Could you check a few things on this model? Use its own coordinates, in mm. Give positions to 0.01 mm unless a question says otherwise; leave off trailing zeros. Loops run counter-clockwise (first coordinate to the right, second up) from the corner with the lowest first, then second, coordinate; pieces in that order, holes last. Notation, with made-up numbers: (2, 11.5) - (22, 11.5) arc R33 ccw to (22, 46.5) - close; hole circle Ø11 at (-10, 20.5). An arc over 180 degrees is marked (long way). Write each question's results on one line, items separated by ' | '. Start each with the question number.
1) If I drill on probe 1 along X at (y, z) = (1, -38.25); probe 2 along Z at (x, y) = (38.5, 3.45); probe 3 along X at (y, z) = (2.4, -18), over which ranges is the centre line in solid material (lowest first)? Write a range as [from, to].
2) I want a section at A-A, the plane z = 0. Write out the boundary of the cut face in (x, y).
3) I want a section at D-D, the plane y = 2.15. Count the separate pieces of the cut face and the enclosed holes in it, and give its area (3 significant figures).
4) I want a section at C-C, the plane x = 2. Write out the boundary of the cut face in (y, z).
5) I want a section at B-B, the plane z = -38.25. Write out the boundary of the cut face in (x, y), and give its area (3 significant figures).
6) If we mould it in two halves opening along X, with no side actions, what happens to faces 1 (the face through (-1, 5, -11)), 2 (the face through (15, 2, 0))? For each: +X half, -X half, draft (parallel to the pull), parting line (faces both ways), or undercut.
from build123d import *

# Parameters (mm, degrees)
SKETCH1_W               = 90
SKETCH1_H               = 90
SKETCH1_R               = 3.501345848
BOSS_EXTRUDE1_DEPTH     = 5
SKETCH2_R               = 1.75
SKETCH2_W               = 5
SKETCH2_H               = 10
CUT_EXTRUDE1_DEPTH      = 1
CUT_EXTRUDE1_DEPTH_BACK = 6
SKETCH3_R               = 4
CUT_EXTRUDE2_DEPTH      = 10


with BuildPart() as part:
    # Sketch1 → Boss-Extrude1 (new body)
    with BuildSketch(Plane(origin=(0, 0, 0), x_dir=(1, 0, 0), z_dir=(0, 1, 0))):
        Rectangle(SKETCH1_W, SKETCH1_H)
        Circle(SKETCH1_R, mode=Mode.SUBTRACT)
        with BuildLine():
            Line((-26.585786438, 19.514718626), (-14.489985056, 7.418917244))
            ThreePointArc((-14.489985056, 7.418917244), (-13.949056578, 6.425915745), (-14.033116428, 5.298267955))
            ThreePointArc((-14.033116428, 5.298267955), (-15, 0), (-14.033116428, -5.298267955))
            ThreePointArc((-14.033116428, -5.298267955), (-13.949056578, -6.425915745), (-14.489985056, -7.418917244))
            Line((-14.489985056, -7.418917244), (-26.585786438, -19.514718626))
            ThreePointArc((-26.585786438, -19.514718626), (-28.765366865, -19.948264128), (-30, -18.100505063))
            Line((-30, -18.100505063), (-30, 18.100505063))
            ThreePointArc((-30, 18.100505063), (-28.765366865, 19.948264128), (-26.585786438, 19.514718626))
        make_face(mode=Mode.SUBTRACT)
        with BuildLine():
            Line((-18.100505063, 30), (18.100505063, 30))
            ThreePointArc((18.100505063, 30), (19.948264128, 28.765366865), (19.514718626, 26.585786438))
            Line((19.514718626, 26.585786438), (7.418917244, 14.489985056))
            ThreePointArc((7.418917244, 14.489985056), (6.425915745, 13.949056578), (5.298267955, 14.033116428))
            ThreePointArc((5.298267955, 14.033116428), (0, 15), (-5.298267955, 14.033116428))
            ThreePointArc((-5.298267955, 14.033116428), (-6.425915745, 13.949056578), (-7.418917244, 14.489985056))
            Line((-7.418917244, 14.489985056), (-19.514718626, 26.585786438))
            ThreePointArc((-19.514718626, 26.585786438), (-19.948264128, 28.765366865), (-18.100505063, 30))
        make_face(mode=Mode.SUBTRACT)
        with BuildLine():
            Line((30, 18.100505063), (30, -18.100505063))
            ThreePointArc((30, -18.100505063), (28.765366865, -19.948264128), (26.585786438, -19.514718626))
            Line((26.585786438, -19.514718626), (14.489985056, -7.418917244))
            ThreePointArc((14.489985056, -7.418917244), (13.949056578, -6.425915745), (14.033116428, -5.298267955))
            ThreePointArc((14.033116428, -5.298267955), (15, 0), (14.033116428, 5.298267955))
            ThreePointArc((14.033116428, 5.298267955), (13.949056578, 6.425915745), (14.489985056, 7.418917244))
            Line((14.489985056, 7.418917244), (26.585786438, 19.514718626))
            ThreePointArc((26.585786438, 19.514718626), (28.765366865, 19.948264128), (30, 18.100505063))
        make_face(mode=Mode.SUBTRACT)
        with BuildLine():
            Line((19.514718626, -26.585786438), (7.418917244, -14.489985056))
            ThreePointArc((7.418917244, -14.489985056), (6.425915745, -13.949056578), (5.298267955, -14.033116428))
            ThreePointArc((5.298267955, -14.033116428), (0, -15), (-5.298267955, -14.033116428))
            ThreePointArc((-5.298267955, -14.033116428), (-6.425915745, -13.949056578), (-7.418917244, -14.489985056))
            Line((-7.418917244, -14.489985056), (-19.514718626, -26.585786438))
            ThreePointArc((-19.514718626, -26.585786438), (-19.948264128, -28.765366865), (-18.100505063, -30))
            Line((-18.100505063, -30), (18.100505063, -30))
            ThreePointArc((18.100505063, -30), (19.948264128, -28.765366865), (19.514718626, -26.585786438))
        make_face(mode=Mode.SUBTRACT)
    extrude(amount=BOSS_EXTRUDE1_DEPTH)

    # Sketch2 → Cut-Extrude1 (cut, two sides)
    with BuildSketch(Plane(origin=(0, 5, 0), x_dir=(1, 0, 0), z_dir=(0, 1, 0))) as cut_extrude1_sk:
        with Locations((-30, -38.25)):
            Circle(SKETCH2_R)
        with Locations((30, -38.25)):
            Circle(SKETCH2_R)
        with Locations((30, 38.25)):
            Circle(SKETCH2_R)
        with Locations((-30, 38.25)):
            Circle(SKETCH2_R)
        with Locations((37.5, 25)):
            Rectangle(SKETCH2_W, SKETCH2_H)
        with Locations((37.5, -25)):
            Rectangle(SKETCH2_W, SKETCH2_H)
        with Locations((-37.5, -25)):
            Rectangle(SKETCH2_W, SKETCH2_H)
        with Locations((-37.5, 25)):
            Rectangle(SKETCH2_W, SKETCH2_H)
    extrude(amount=CUT_EXTRUDE1_DEPTH, mode=Mode.SUBTRACT)
    extrude(cut_extrude1_sk.sketch, amount=-CUT_EXTRUDE1_DEPTH_BACK, mode=Mode.SUBTRACT)

    # Sketch3 → Cut-Extrude2 (cut)
    with BuildSketch(Plane(origin=(0, 5, 0), x_dir=(1, 0, 0), z_dir=(0, 1, 0))):
        Circle(SKETCH3_R)
    extrude(amount=-CUT_EXTRUDE2_DEPTH, mode=Mode.SUBTRACT)


solid = part.part
Answers:
1) probe 1: x = [-45, -31.75], [-28.25, 28.25], [31.75, 45] | probe 2: z = [-45, -30], [-20, 20], [30, 45] | probe 3: x = [-45, -30], [-25.07, -10.93], [10.93, 25.07], [30, 45]
2) outline: (-45, 0) - (-30, 0) - (-30, 5) - (-45, 5) - close; (-15, 0) - (-4, 0) - (-4, 5) - (-15, 5) - close; (4, 0) - (15, 0) - (15, 5) - (4, 5) - close; (30, 0) - (45, 0) - (45, 5) - (30, 5) - close
3) separate pieces: 1 | enclosed holes: 13 | area: 5,970 mm2
4) outline: (0, -45) - (5, -45) - (5, -30) - (0, -30) - close; (0, -14.87) - (5, -14.87) - (5, -3.46) - (0, -3.46) - close; (0, 3.46) - (5, 3.46) - (5, 14.87) - (0, 14.87) - close; (0, 30) - (5, 30) - (5, 45) - (0, 45) - close
5) outline: (-45, 0) - (-31.75, 0) - (-31.75, 5) - (-45, 5) - close; (-28.25, 0) - (28.25, 0) - (28.25, 5) - (-28.25, 5) - close; (31.75, 0) - (45, 0) - (45, 5) - (31.75, 5) - close | area: 415 mm2
6) face 1: draft | face 2: undercut
